Check sheet for the drawn part. Datum: minimum x, y, z corner. Units: mm. Round coordinates to 2 decimals unless told otherwise and drop trailing zeros. Loops run counter-clockwise (first coordinate to the right, second up) from the corner with the lowest first, then second, coordinate; pieces in that order, holes last.
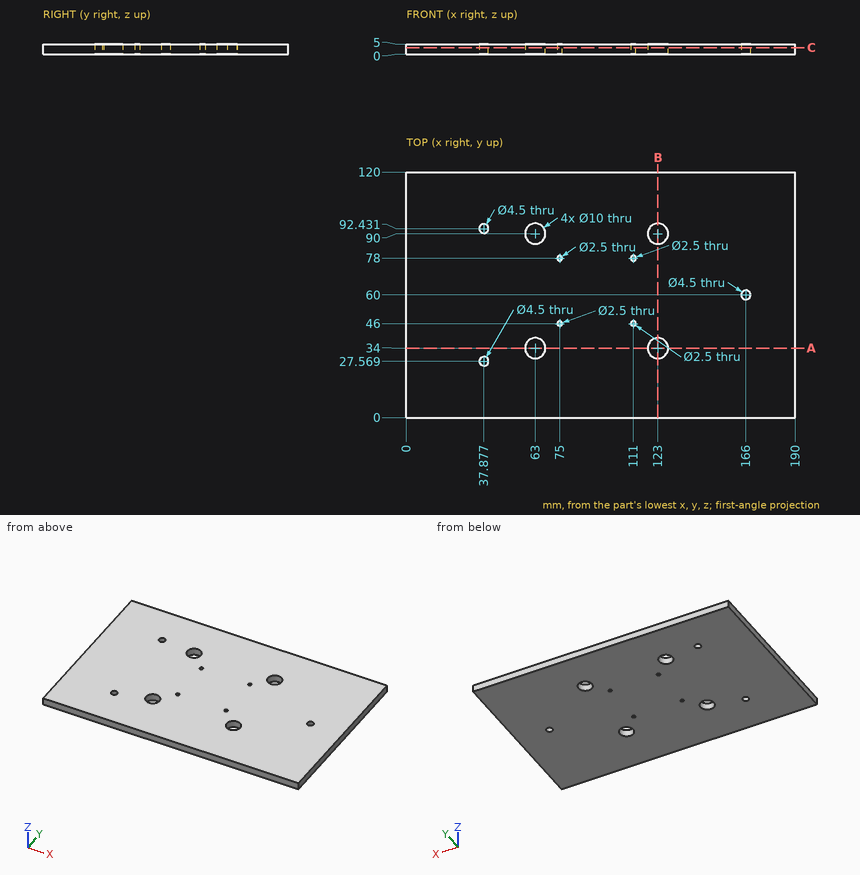
1) Sectioned sample at C-C, the plane z = 3.25. State how many separate pieces and enclosed holes the cut face has, then the cut area to 3 significant figures.
Report:
separate pieces: 1
enclosed holes: 11
area: 22,400 mm2
2) Sectioned sample at A-A, the plane y = 34. Record the cut outline in (x, z).
Report:
outline: (0, 0) - (58, 0) - (58, 5) - (0, 5) - close; (68, 0) - (118, 0) - (118, 5) - (68, 5) - close; (128, 0) - (190, 0) - (190, 5) - (128, 5) - close
3) Scan lines: line 1 along Y through (x, z) = (75, 1.75); line 2 along X through (y, z) = (34.5, 0.8) (1 decimal); line 3 along X through (y, z) = (46, 3.7). Record each from-to range of solid material in increasing order.
Report:
line 1: y = 0 to 44.75, 47.25 to 76.75, 79.25 to 120
line 2: x = 0 to 58, 68 to 118, 128 to 190
line 3: x = 0 to 73.75, 76.25 to 109.75, 112.25 to 190
4) Sectioned sample at B-B, the plane x = 123. Record the cut outline in (y, z).
Report:
outline: (0, 0) - (29, 0) - (29, 5) - (0, 5) - close; (39, 0) - (85, 0) - (85, 5) - (39, 5) - close; (95, 0) - (120, 0) - (120, 5) - (95, 5) - close
